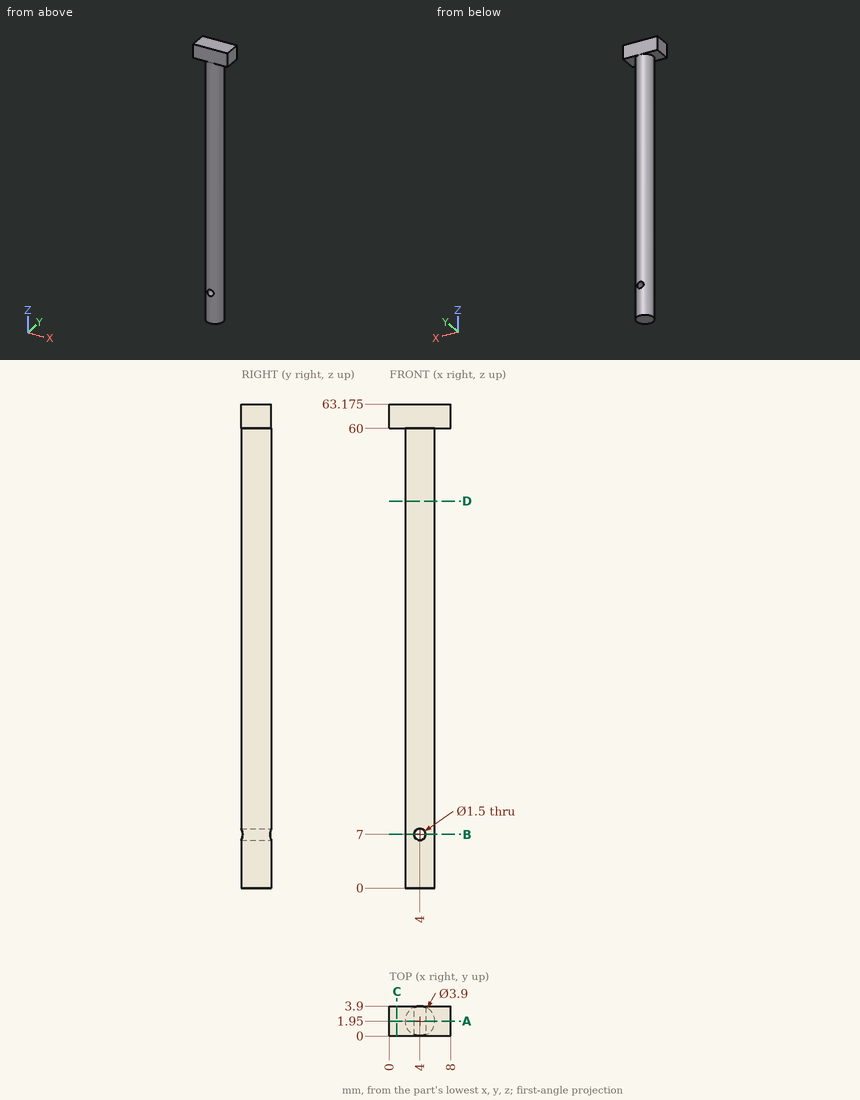
Verification items for this drawing (mm, ordinates from the low corner). Coordinates: 2 decimals unless noted, no trailing zeros. Order: outer loops, then holes, each group sorted by start corner. A loop starts at its lowest first (then second) coordinate and runs counter-clockwise, first axis right, second up. Notation, with made-up numbers: M -0.5,78.5 L 29.5,78.5 A14 cw 29.5,86.5 Z; hole C 56,17 d9. An arc over 180 degrees is marked long. One line per item, written item: value. Start each with the question number.
Item 1: Sectioned sample at B-B on z = 7. Record the cut outline in (x, y).
Item 2: Thickness scan on probe 1 along Z at (x, y) = (4, 0.8) (3 decimals); probe 2 along Z at (x, y) = (6.25, 3.3) (3 decimals); probe 3 along Z at (x, y) = (3.5, 2.55) (3 decimals). Record the ranges inside material, lowest first.
Item 3: Sectioned sample at A-A on y = 1.95. Record the cut outline in (x, z) (3 decimals), then the cut area to 3 significant figures.
Item 4: Sectioned sample at D-D on z = 50.5. Record the cut outline in (x, y), then the cut area to 3 significant figures.
Item 5: Sectioned sample at C-C on x = 1. Record the cut outline in (y, z) (3 decimals), then the cut area to 3 significant figures.
Calculated:
1. outline: M 3.25,0.15 L 3.25,3.75 A1.95 ccw Z; M 4.75,0.15 A1.95 ccw 4.75,3.75 Z
2. probe 1: 0 to 6.25, 7.75 to 63.175
2. probe 2: 60 to 63.175
2. probe 3: 0 to 6.441, 7.559 to 63.175
3. outline: M 0,60 L 2.05,60 L 2.05,0 L 5.95,0 L 5.95,60 L 8,60 L 8,63.175 L 0,63.175 Z; hole C 4,7 d1.5
3. area: 258 mm^2
4. outline: C 4,1.95 d3.9
4. area: 11.9 mm^2
5. outline: M 0,60 L 3.9,60 L 3.9,63.175 L 0,63.175 Z
5. area: 12.4 mm^2
